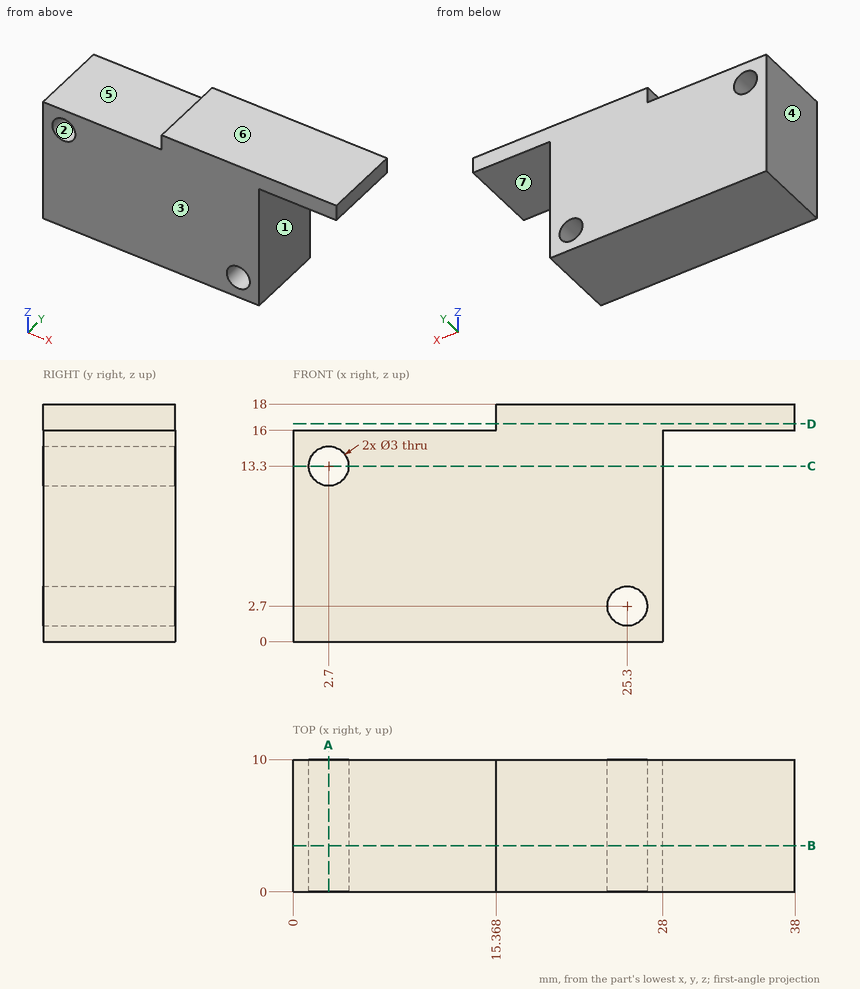
Part print with two shaded views. Sizes in mm from the minimum x, y, z corner. A direction names the side the tool comes from. Coordinates: 2 decimals unless noted, no trailing zeros. Loops run counter-clockwise (first coordinate to the right, second up) from the corner with the lowest first, then second, coordinate; pieces in that order, holes last. Notation, with made-up numbers: (-37, -6.75) - (9, -6.75) arc R19 cw to (9, 19.25) - close; hole circle Ø10 at (9, 40.5). An arc over 180 degrees is marked (long way). Write each question's results on one line, items separated by ' | '. Start each with the question number.
Q1. Slice it at D-D on z = 16.5. Give the cut face in (x, y), and give its area (3 significant figures).
Q2. Probe line 1 along X through (y, z) = (2.25, 2.7); line 2 along Z through (x, y) = (2.7, 4.75); line 3 along Z through (x, y) = (25.3, 3.5). List the from-to ranges inside material, lowest first.
Q3. Slice it at A-A on x = 2.7. Give the cut face in (y, z).
Q4. Slice it at B-B on y = 3.5. Give the cut face in (x, z), and give its area (3 significant figures).
Q5. Which spindle directions (+Z, -Z, +X, -X, +Y, -Y) get a long thin tool onto all of the face, cutting with end or side? Do the marked faces 5, 6 and 7. Say none if no direction does.
Q6. Drop flat-ended pins along their axis: pin 1 Ø5 at (x, y) = (7, 2.5) entering from +Z; pin 2 Ø1.6 at (y, z) = (3, 17) entering from -X; pin 3 Ø3 at (y, z) = (3, 4) entering from +X. Give the stop position or say it passes through.
Q7. Two-plate mould, pull along X, no slides. Class the marked faces 1, 2, 3 and 4: +X half, -X half, draft (parallel to the pull), parting line (faces both ways), or undercut.
Q8. Slice it at C-C on z = 13.3. Give the cut face in (x, y).
Answer:
1) outline: (15.37, 0) - (38, 0) - (38, 10) - (15.37, 10) - close | area: 226 mm2
2) line 1: x = 0 to 23.8, 26.8 to 28 | line 2: z = 0 to 11.8, 14.8 to 16 | line 3: z = 0 to 1.2, 4.2 to 18
3) outline: (0, 0) - (10, 0) - (10, 11.8) - (0, 11.8) - close; (0, 14.8) - (10, 14.8) - (10, 16) - (0, 16) - close
4) outline: (0, 0) - (28, 0) - (28, 16) - (38, 16) - (38, 18) - (15.37, 18) - (15.37, 16) - (0, 16) - close; hole circle Ø3 at (2.7, 13.3); hole circle Ø3 at (25.3, 2.7) | area: 479 mm2
5) face 5: +Z, -X, +Y, -Y | face 6: +Z, +X, -X, +Y, -Y | face 7: -Z, +X, +Y, -Y
6) pin 1: stops at z = 16 | pin 2: stops at x = 15.37 | pin 3: stops at x = 28
7) face 1: +X half | face 2: undercut | face 3: draft | face 4: -X half
8) outline: (0, 0) - (1.2, 0) - (1.2, 10) - (0, 10) - close; (4.2, 0) - (28, 0) - (28, 10) - (4.2, 10) - close
